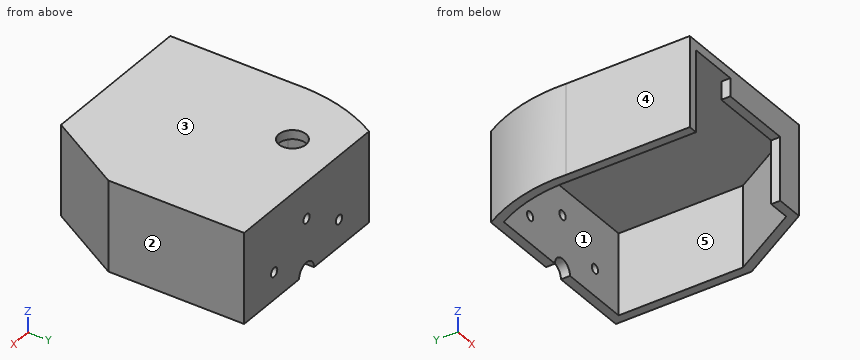
Autodesk Inventor part; units mm, degrees
ref_plane "YZ Plane" through (0, 0, 0) normal (1, 0, 0) x (0, 1, 0)
ref_plane "XZ Plane" through (0, 0, 0) normal (0, 1, 0) x (-1, 0, 0)
ref_plane "XY Plane" through (0, 0, 0) normal (0, 0, 1) x (1, 0, 0)
sketch "Sketch1" plane through (0, 0, 0) normal (0, 0, 1) x (1, 0, 0)
  line L0 (0, 0) -> (100, 0)
  line L1 (100, 0) -> (100, -75)
  line L2 (100, -75) -> (75, -118.3013)
  line L3 (75, -118.3013) -> (-12.5, -118.3013)
  line L4 (-12.5, -118.3013) -> (-12.5, -50)
  arc A0 (0, 0) -> (-12.5, -50) centre (77.4072, -45.9143) ccw
  dimension "d0" = 100
  dimension "d1" = 75
  dimension "d2" = 50
  dimension "d3" = 150
  dimension "d5" = 50
  dimension "d6" = 12.5
  dimension "d7" = 90
extrude "Extrusion1" add sketch "Sketch1" along normal blind 50
sketch "Sketch2" plane through (0, 0, 0) normal (0, 0, -1) x (-1, 0, 0)
  line L0 (0, 0) -> (-100, 0)
  line L1 (-100, 0) -> (-100, -75)
  line L2 (-100, -75) -> (-75, -118.3013)
  line L3 (-75, -118.3013) -> (12.5, -118.3013)
  line L4 (12.5, -118.3013) -> (12.5, -50)
  arc A0 (12.5, -50) -> (0, 0) centre (-77.4072, -45.9143) ccw
  line L5 (-95, -73.6603) -> (-95, -5)
  line L6 (-95, -5) -> (-2.902, -5)
  arc A1 (7.5, -49.8848) -> (-2.902, -5) centre (-77.4072, -45.9143) ccw
  line L7 (7.5, -49.8848) -> (7.5, -113.3013)
  line L8 (7.5, -113.3013) -> (-72.1132, -113.3013)
  line L9 (-72.1132, -113.3013) -> (-95, -73.6603)
  dimension "d10" = 5
extrude "Extrusion2" cut sketch "Sketch2" against normal blind 45 contours L5 L6 A1 L7 L8 L9
sketch "Sketch3" plane through (0, 0, 0) normal (0, 0, -1) x (-1, 0, 0)
  line L0 (7.5, -113.3013) -> (-72.1132, -113.3013)
  line L1 (12.5, -118.3013) -> (-75, -118.3013)
  line L2 (7.5, -113.3013) -> (-60, -113.3013)
  line L3 (-60, -113.3013) -> (-60, -118.3013)
  line L4 (-60, -118.3013) -> (7.5, -118.3013)
  line L5 (7.5, -118.3013) -> (7.5, -113.3013)
  point P0 (0, 0)
  dimension "d13" = 15
extrude "Extrusion3" cut sketch "Sketch3" against normal blind 45
sketch "Sketch4" plane through (0, 0, 0) normal (0, 1, 0) x (1, 0, 0)
  circle A0 centre (50, 0) radius 6
  line L0 (0, 0) -> (100, 0)
  dimension "d16" = 12
extrude "Extrusion4" cut sketch "Sketch4" against normal through all
sketch "Sketch5" plane through (0, 0, 50) normal (0, 1, 0) x (1, 0, 0)
  arc A0 (44, 50) -> (56, 50) centre (50, 50) ccw
  circle A1 centre (50, 50) radius 30 construction
  circle A2 centre (50, 20) radius 2.5
  circle A3 centre (75.9808, 35) radius 2.5
  circle A4 centre (75.9808, 65) radius 2.5
  circle A5 centre (50, 80) radius 2.5
  circle A6 centre (24.0192, 65) radius 2.5
  circle A7 centre (24.0192, 35) radius 2.5
  point P0 (0, 50)
  dimension "d19" = 60
  dimension "d20" = 5
  dimension "d23" = 360
extrude "Extrusion5" cut sketch "Sketch5" against normal blind 5 contours A2 | A3 | A7
sketch "Sketch6" plane through (0, 0, 50) normal (0, 0, 1) x (1, 0, 0)
  circle A0 centre (25, -25) radius 7.5
  point P0 (0, 0)
  dimension "d27" = 15
  dimension "d28" = 25
  dimension "d29" = 25
extrude "Extrusion6" cut sketch "Sketch6" against normal blind 5
sketch "Sketch7" plane through (-12.5, -118.3013, 50) normal (0, -1, 0) x (1, 0, 0)
  line L0 (87.5, 0) -> (112.5, 0)
  line L1 (87.5, 0) -> (32.5, 0)
  line L2 (32.5, 0) -> (32.5, -15)
  line L3 (32.5, -15) -> (87.5, -15)
  line L4 (87.5, -15) -> (87.5, 0)
  line L5 (0, -50) -> (0, 0)
  point P0 (12.5, -50)
  dimension "d32" = 15
  dimension "d33" = 32.5
extrude "Extrusion7" add sketch "Sketch7" against normal blind 5
properties part number "FA002" material "ABS Plastic"
Read the model definition and answer for the solid it produces. Units are mm, in the model's axes. Face numbers are marked on the shaded views. A direction names the side the tool comes from. Round coordinates to 2 decimals unless told otherwise and drop trailing zeros. Write each loop counter-clockwise with the first axis right and the second up, starting at its lowest first coordinate (ties: lowest second). Pieces come first, ordered by that corner, then holes. Notation, with made-up numbers: (56.5, 62) - (78.5, 62) arc R17 ccw to (78.5, 81) - close; hole circle Ø4 at (68.25, 16.5). An arc over 180 degrees is marked (long way). Use CSV: the item, a comma, the result in double quotes.
Q1. Find section B-B, the plane y = -25. Write down the section's boundary in (x, z), then the cut area to 3 significant figures.
Values:
outline,"(-10.13, 0) - (-4.98, 0) - (-4.98, 45) - (17.5, 45) - (17.5, 50) - (-10.13, 50) - close; (32.5, 45) - (95, 45) - (95, 0) - (100, 0) - (100, 50) - (32.5, 50) - close"
area,"932 mm²"
Q2. Determine the mould class of the marked faces 3, 4 and 5 for opening direction X: +X half, -X half, draft (parallel to the pull), parting line (faces both ways), or undercut.
Values:
face 3,"draft"
face 4,"-X half"
face 5,"undercut"
Q3. Find section D-D, the plane x = 45.5. Write down the section's boundary in (y, z), then the cut area to 3 significant figures.
Values:
outline,"(-118.3, 35) - (-113.3, 35) - (-113.3, 45) - (-5, 45) - (-5, 3.97) - (0, 3.97) - (0, 50) - (-118.3, 50) - close"
area,"847 mm²"
Q4. Straight lines are drawn through the part: line 1 along X through (y, z) = (-65, 42.5); line 2 along X through (y, z) = (-3.6, 15); line 3 along Y through (x, z) = (25, 46.8). For each, find the intervals that lie inside material, in ascending order.
Values:
line 1,"x = -12.5 to -7.5, 95 to 100"
line 2,"x = -2.03 to 21.52, 26.52 to 73.48, 78.48 to 100"
line 3,"y = -118.3 to -32.5, -17.5 to 0"
Q5. Find section A-A, the plane z = 15. Write down the section's boundary in (x, y).
Values:
outline,"(-12.5, -118.3) - (-7.5, -118.3) - (-7.5, -49.88) arc R85 cw to (2.9, -5) - (21.52, -5) - (21.52, 0) - (0, 0) arc R90 ccw to (-12.5, -50) - close; (26.52, -5) - (73.48, -5) - (73.48, 0) - (26.52, 0) - close; (60, -118.3) - (75, -118.3) - (100, -75) - (100, 0) - (78.48, 0) - (78.48, -5) - (95, -5) - (95, -73.66) - (72.11, -113.3) - (60, -113.3) - close"
Q6. A tool of negligible diameter and unlimited length cuts with its end or side. For the marked faces 1 and 2, from which of +Z, -Z, +X, -X, +Y, -Y can it reach the whole face along a straight path? Write none if from no direction.
Values:
face 1,"-Z"
face 2,"+Z, -Z, +X, +Y, -Y"
Q7. Find section C-C, the plane z = 30. Write down the section's boundary in (x, y).
Values:
outline,"(-12.5, -118.3) - (-7.5, -118.3) - (-7.5, -49.88) arc R85 cw to (2.9, -5) - (47.5, -5) - (47.5, 0) - (0, 0) arc R90 ccw to (-12.5, -50) - close; (52.5, -5) - (95, -5) - (95, -73.66) - (72.11, -113.3) - (60, -113.3) - (60, -118.3) - (75, -118.3) - (100, -75) - (100, 0) - (52.5, 0) - close"
Q8. Each of these flat-tipped pins is pushed along its axis until it touches: pin 1 Ø6 at (x, y) = (44, -41) entering from -Z; pin 2 Ø13.5 at (y, z) = (-26, 18) entering from -X; pin 3 Ø5 at (y, z) = (-96.5, 24.5) entering from +X. Where does it stop, or does it pass through?
Values:
pin 1,"stops at z = 45"
pin 2,"stops at x = -11.62"
pin 3,"stops at x = 89.03"
